For this review, take the finished solid that the model builds, in its own axes (mm). A direction names the side the tool comes from. Coordinates: 2 decimals unless noted, no trailing zeros. Write each loop counter-clockwise with the first axis right and the second up, starting at its lowest first coordinate (ties: lowest second). Pieces come first, ordered by that corner, then holes.
1) We need section C-C on y = 0.5. Write out the cut boundary in (x, z).
2) We need section D-D on y = -12.5. Write out the cut boundary in (x, z).
3) Mouldability with a two-part tool opening along Y and no side actions: class faces 1 (the face through (10.73, -5.84, 2.26)), 2 (the face through (-10, 2.5, 1)), 3 (the face through (-20.2, -5, 1)) as pulls with the +Y half, pulls with the -Y half, needs draft (parallel to the pull), parting line crosses it, or undercut.
4) To check wall thickness, follow line 1 along X through (y, z) = (-17, 2.35); line 2 along Y through (x, z) = (-2.5, 1.8); line 3 along X through (y, z) = (0.5, 2.2). State the ranges of each line that lie inside material, in increasing order.
5) We need section B-B on x = 11.8. Write out the cut boundary in (y, z).
6) Insertion check: P1, Ø0.7, axis at x = 0.5, z = 1.5, coming from the +Y side; P2, Ø6, axis at x = -15, y = -17, coming from the -Z side; P3, Ø1.6, axis at x = -7, z = 2, coming from the -Y side; P4, Ø1, axis at y = -16.5, z = 2.5, coming from the -X side. Each pin has a flat end and moves straight along its axis. Give the tip position at first contact, or say it passes through.
7) For faces 4 (the face through (-0.2, 1, 1)), 5 (the face through (11.73, -4.86, 2.26)), 6 (the face through (-17, 0, 2)), list the 3-axis set-ups (+Z, -Z, +X, -X, +Y, -Y) from which the entire face can be reached by the end or side of a thin tool; tool diameter is ignored.
Autodesk Inventor part; units mm, degrees
ref_plane "YZ Plane" through (0, 0, 0) normal (1, 0, 0) x (0, 1, 0)
ref_plane "XZ Plane" through (0, 0, 0) normal (0, 1, 0) x (-1, 0, 0)
ref_plane "XY Plane" through (0, 0, 0) normal (0, 0, 1) x (1, 0, 0)
sketch "Эскиз1" plane through (0, 0, 0) normal (0, 0, 1) x (1, 0, 0)
  line L0 (-0.2, 0) -> (-0.2, 2.5)
  line L1 (-0.2, 2.5) -> (-20.2, 2.5)
  line L2 (-20.2, 0) -> (-20.2, 2.5)
  line L3 (-0.2, 0) -> (1.2, 0)
  line L4 (1.2, 0) -> (1.2, -3.5)
  line L5 (-20.2, -13) -> (-17.2, -13)
  line L6 (-17.2, -7) -> (7.8, -7)
  line L7 (7.8, -13) -> (15.8, -13)
  line L8 (15.8, -3.5) -> (1.2, -3.5)
  line L9 (7.8, -13) -> (7.8, -17)
  line L10 (15.8, -17) -> (15.8, -13)
  arc A0 (7.8, -17) -> (15.8, -17) centre (11.8, -17) ccw
  circle A1 centre (11.8, -17) radius 1.25
  line L11 (15.8, -13) -> (15.8, -3.5)
  line L12 (7.8, -7) -> (7.8, -13)
  line L13 (-17.2, -7) -> (-17.2, -13)
  line L14 (-20.2, -13) -> (-20.2, 0)
  line L15 (-6.1183, 2.5) -> (-8.8117, 2.5)
  point P0 (0, 0)
  dimension "d0" = 2.5
extrude "Выдавливание1" add sketch "Эскиз1" along normal blind 3
sketch "Эскиз2" plane through (1.2, -3.5, 0) normal (0, 1, 0) x (1, 0, 0)
  line L0 (11.85, 0) -> (11.85, -3)
  line L1 (14.6, 0) -> (0, 0)
  line L2 (0, 0) -> (0, -3)
  line L3 (14.6, -3) -> (0, -3)
  line L4 (14.6, 0) -> (14.6, -3)
  point P0 (-1.2, 0)
extrude "Выдавливание2" add sketch "Эскиз2" along normal blind 1
fillet "Сопряжение1" radius 2 2 edges at (15.8, -2.5, 1.5) (1.2, -2.5, 1.5)
fillet "Сопряжение1" radius 1.5 2 edges at (-17.2, -13, 1.5) (-20.2, -13, 1.5)
sketch "Эскиз3" plane through (0, 0, 3) normal (0, 0, 1) x (1, 0, 0)
  line L0 (-18.4, 2.5) -> (-18.4, -2.75)
  arc A0 (-18.4, -2.75) -> (-15.7, -5.45) centre (-15.7, -2.75) ccw
  line L1 (-15.7, -5.45) -> (9.8, -5.45)
  arc A1 (11.1, -6.75) -> (9.8, -5.45) centre (9.8, -6.75) ccw
  line L2 (11.1, -6.75) -> (11.1, -15.75)
  line L3 (12.5, -15.75) -> (12.5, -6.75)
  arc A2 (12.5, -6.75) -> (9.8, -4.05) centre (9.8, -6.75) ccw
  line L4 (9.8, -4.05) -> (-15.7, -4.05)
  arc A3 (-17, -2.75) -> (-15.7, -4.05) centre (-15.7, -2.75) ccw
  line L5 (-17, -2.75) -> (-17, 2.5)
  line L6 (-17, 2.5) -> (-18.4, 2.5)
  line L7 (12.5, -15.75) -> (12.5, -17.0201)
  line L8 (12.5, -17.0201) -> (11.1, -17.0201)
  line L9 (11.1, -17.0201) -> (11.1, -15.75)
  point P0 (0, 0)
extrude "Выдавливание3" cut sketch "Эскиз3" against normal blind 1.5
properties part number "RackeSecondaryStacring"
Result:
1. outline: (-20.2, 0) - (-0.2, 0) - (-0.2, 3) - (-17, 3) - (-17, 1.5) - (-18.4, 1.5) - (-18.4, 3) - (-20.2, 3) - close
2. outline: (-19.82, 0) - (-17.58, 0) - (-17.58, 3) - (-19.82, 3) - close; (7.8, 0) - (15.8, 0) - (15.8, 3) - (12.5, 3) - (12.5, 1.5) - (11.1, 1.5) - (11.1, 3) - (7.8, 3) - close
3. face 1: undercut
3. face 2: pulls with the +Y half
3. face 3: needs draft
4. line 1: x = 7.8 to 10.55, 13.05 to 15.8
4. line 2: y = -7 to -5.45, -4.05 to 2.5
4. line 3: x = -20.2 to -18.4, -17 to -0.2
5. outline: (-21, 0) - (-18.25, 0) - (-18.25, 3) - (-21, 3) - close; (-15.75, 0) - (-2.5, 0) - (-2.5, 3) - (-4.94, 3) - (-4.94, 1.5) - (-15.75, 1.5) - close
6. P1: stops at y = 0
6. P2: passes through
6. P3: stops at y = -7
6. P4: stops at x = 7.8
7. face 4: +Z, -Z, +X, +Y
7. face 5: +Z
7. face 6: +Z, +Y
